Autodesk Inventor part; units mm, degrees
ref_plane "YZ Plane" through (0, 0, 0) normal (1, 0, 0) x (0, 1, 0)
ref_plane "XZ Plane" through (0, 0, 0) normal (0, 1, 0) x (-1, 0, 0)
ref_plane "XY Plane" through (0, 0, 0) normal (0, 0, 1) x (1, 0, 0)
sketch "Sketch1" plane through (0, 0, 0) normal (0, 1, 0) x (-1, 0, 0)
  line L0 (-57.5, 21.5) -> (57.5, 21.5)
  line L1 (57.5, 21.5) -> (57.5, -21.5)
  line L2 (57.5, -21.5) -> (-57.5, -21.5)
  line L3 (-57.5, -21.5) -> (-57.5, 21.5)
  line L4 (-57.5, 21.5) -> (57.5, -21.5) construction
  line L5 (57.5, 21.5) -> (-57.5, -21.5) construction
  point P0 (0, 0)
  dimension "d0" = 115
  dimension "d1" = 43
extrude "Extrusion1" add sketch "Sketch1" along normal blind 1.6
sketch "Sketch2" plane through (0, 1.6, 0) normal (0, 1, 0) x (1, 0, 0)
  line L0 (57.5, 21.5) -> (-57.5, 21.5)
  line L1 (57.5, 21.5) -> (54.5, 21.5)
  line L2 (57.5, -21.5) -> (57.5, 21.5)
  line L3 (54.5, 21.5) -> (57.5, 21.5)
  line L4 (57.5, 21.5) -> (57.5, 18.5)
  line L5 (57.5, 18.5) -> (54.5, 21.5)
  point P0 (0, 0)
  dimension "d4" = 3
  dimension "d5" = 3
extrude "Extrusion2" cut sketch "Sketch2" against normal blind 1.6
sketch "Sketch3" plane through (0, 1.6, 0) normal (0, 1, 0) x (1, 0, 0)
  line L0 (57.5, -21.5) -> (57.5, 18.5)
  circle A0 centre (53.5, 17.5) radius 1.5
  point P0 (0, 0)
  dimension "d11" = 3
extrude "Extrusion3" cut sketch "Sketch3" against normal blind 1.6
sketch "Sketch4" plane through (0, 1.6, 0) normal (0, 1, 0) x (1, 0, 0)
  line L0 (-57.5, 21.5) -> (-57.5, -21.5)
  line L1 (-57.5, 15) -> (-49.5, 15)
  line L2 (-49.5, 15) -> (-49.5, 18.5)
  line L3 (54.5, 21.5) -> (-57.5, 21.5)
  line L4 (-46.5, 21.5) -> (-49.5, 18.5)
  circle A0 centre (-45.5, 18) radius 1.5
  point P0 (0, 0)
  dimension "d15" = 8
  dimension "d16" = 3.5
  dimension "d20" = 3
extrude "Extrusion4" cut sketch "Sketch4" against normal blind 1.6 contours L3 L4 L2 L1 L0
sketch "Sketch5" plane through (0, 1.6, 0) normal (0, 1, 0) x (1, 0, 0)
  line L0 (54.5, 21.5) -> (-46.5, 21.5)
  circle A0 centre (-45.5, 17.5) radius 1.5
  point P0 (0, 0)
  dimension "d25" = 3
extrude "Extrusion5" cut sketch "Sketch5" against normal blind 1.6
mirror "Mirror1" about plane through (0, 0, 0) normal (0, 0, 1) of "Extrusion4", "Extrusion5", "Extrusion2"
sketch "Sketch7" plane through (0, 1.6, 0) normal (0, 1, 0) x (1, 0, 0)
  line L0 (-54.4988, 14.0073) -> (-26.4988, 14.0073)
  line L1 (-26.4988, 14.0073) -> (-26.4988, -13.9927)
  line L2 (-26.4988, -13.9927) -> (-54.4988, -13.9927)
  line L3 (-54.4988, -13.9927) -> (-54.4988, 14.0073)
  point P0 (0, 0)
  dimension "d30" = 28
  dimension "d31" = 28
extrude "Extrusion6" add sketch "Sketch7" along normal blind 14
sketch "Sketch8" plane through (0, 15.6, 0) normal (0, 1, 0) x (1, 0, 0)
  line L0 (-26.4988, 14.0073) -> (-26.4988, -13.9927)
  line L1 (-26.4988, 14.0073) -> (-36.4988, 14.0073)
  line L2 (-54.4988, 14.0073) -> (-26.4988, 14.0073)
  line L3 (-36.4988, 14.0073) -> (-37.9988, 14.0073)
  line L4 (-37.9988, 14.0073) -> (-36.4988, 14.0073)
  line L5 (-36.4988, 14.0073) -> (-36.4988, 12.5073)
  line L6 (-36.4988, 12.5073) -> (-48.9988, 12.5073)
  line L7 (-48.9988, 12.5073) -> (-48.9988, -12.4927)
  line L8 (-48.9988, -12.4927) -> (-36.4988, -12.4927)
  line L9 (-36.4988, -12.4927) -> (-36.4988, 12.5073)
  point P0 (0, 0)
  dimension "d34" = 10
  dimension "d35" = 1.5
  dimension "d36" = 1.5
  dimension "d37" = 12.5
  dimension "d38" = 25
extrude "Extrusion7" add sketch "Sketch8" along normal blind 0.2
sketch "Sketch9" plane through (0, 1.6, 0) normal (0, 1, 0) x (1, 0, 0)
  line L0 (-57.5, 15) -> (-57.5, -15)
  line L1 (-57.5, 15) -> (-23.75, 15)
  line L2 (-23.75, 15) -> (-23.75, 5.25)
  line L3 (-23.75, 5.25) -> (-13.25, 5.25)
  line L4 (-13.25, 5.25) -> (-13.25, -5.25)
  line L5 (-13.25, -5.25) -> (-23.75, -5.25)
  line L6 (-23.75, -5.25) -> (-23.75, 5.25)
  point P0 (0, 0)
  dimension "d41" = 33.75
  dimension "d43" = 9.75
  dimension "d44" = 10.5
  dimension "d45" = 10.5
extrude "Extrusion8" add sketch "Sketch9" along normal blind 14
sketch "Sketch10" plane through (0, 15.6, 0) normal (0, 1, 0) x (1, 0, 0)
  circle A0 centre (-18.5, 0) radius 6.25
  point P0 (0, 0)
  dimension "d48" = 12.5
extrude "Extrusion9" add sketch "Sketch10" along normal blind 3.5
sketch "Sketch11" plane through (0, 1.6, 0) normal (0, 1, 0) x (1, 0, 0)
  line L0 (54.5, -21.5) -> (57.5, -18.5)
  line L1 (57.5, -18.5) -> (55.85, -18.5)
  line L2 (55.85, -18.5) -> (55.85, -16.4)
  line L3 (55.85, -16.4) -> (57.5, -16.4)
  line L4 (57.5, -16.4) -> (57.5, -18.5)
  line L5 (55.85, -16.4) -> (-10.35, -16.4)
  line L6 (-10.35, -16.4) -> (-10.35, 3.2)
  line L7 (-10.35, 3.2) -> (55.85, 3.2)
  line L8 (55.85, 3.2) -> (55.85, -16.4)
  point P0 (0, 0)
  dimension "d51" = 1.65
  dimension "d52" = 2.1
  dimension "d53" = 66.2
  dimension "d54" = 19.6
extrude "Extrusion10" add sketch "Sketch11" along normal blind 16 contours L5 L6 L7 L8
sketch "Sketch12" plane through (0, 0, 0) normal (0, -1, 0) x (1, 0, 0)
  line L0 (57.5, 18.5) -> (57.5, -18.5)
  line L1 (57.5, -18.5) -> (57.5, -8.5)
  line L2 (57.5, -8.5) -> (48.2, -8.5)
  line L3 (48.2, -8.5) -> (48.2, 9)
  line L4 (48.2, 9) -> (57.5, 9)
  line L5 (57.5, 9) -> (57.5, -8.5)
  point P0 (0, 0)
  dimension "d57" = 10
  dimension "d58" = 9.3
  dimension "d59" = 17.5
extrude "Extrusion11" add sketch "Sketch12" along normal blind 16
sketch "Sketch13" plane through (0, 0, 0) normal (0, -1, 0) x (1, 0, 0)
  line L0 (57.5, -8.5) -> (48.2, -8.5)
  line L1 (48.2, -8.5) -> (48.2, -16)
  line L2 (48.2, -16) -> (24, -16)
  line L3 (24, -16) -> (24, 9)
  line L4 (24, 9) -> (48.2, 9)
  line L5 (48.2, 9) -> (48.2, -16)
  line L6 (24, -16) -> (24, -20)
  line L7 (54.5, -21.5) -> (-46.5, -21.5)
  line L8 (24, -20) -> (9, -20)
  line L9 (24, 9) -> (24, 10)
  line L10 (24, 10) -> (9, 10)
  line L11 (9, 10) -> (9, -20)
  line L12 (9, -20) -> (24, -20)
  line L13 (24, -20) -> (24, 10)
  point P0 (0, 0)
  dimension "d62" = 7.5
  dimension "d63" = 24.2
  dimension "d64" = 25
  dimension "d65" = 4
  dimension "d66" = 15
  dimension "d67" = 1
extrude "Extrusion12" add sketch "Sketch13" along normal blind 16 contours L1 L2 L3 L4 L5
sketch "Sketch14" plane through (0, 0, 0) normal (0, -1, 0) x (1, 0, 0)
  line L0 (24, -16) -> (24, 9)
  line L1 (24, -16) -> (24, -20)
  line L2 (24, -20) -> (9, -20)
  line L3 (24, 9) -> (24, 10)
  line L4 (24, 10) -> (9, 10)
  line L5 (9, 10) -> (9, -20)
  line L6 (9, -20) -> (24, -20)
  line L7 (24, -20) -> (24, 10)
  point P0 (0, 0)
  dimension "d70" = 4
  dimension "d71" = 15
  dimension "d72" = 1
extrude "Extrusion13" add sketch "Sketch14" along normal blind 27
properties part number "teaser_PCB"
Verification items for the finished model (mm, model axes). A direction names the side the tool comes from. Round coordinates to 2 decimals unless told otherwise and drop trailing zeros. Write each loop counter-clockwise with the first axis right and the second up, starting at its lowest first coordinate (ties: lowest second). Pieces come first, ordered by that corner, then holes. Notation, with made-up numbers: (19, 46.25) -> (44, 46.25) arc R27 cw to (44, 85.25) -> close; hole circle Ø3 at (18, -5). An arc over 180 degrees is marked (long way). Write each question's results on one line, items separated by ' | '.
Q1. Sectioned sample at D-D, the plane x = 38. Record the boundary of the cut face in (y, z), and give its area (3 significant figures).
Derived:
outline: (-16, -16) -> (0, -16) -> (0, -21.5) -> (1.6, -21.5) -> (1.6, -3.2) -> (17.6, -3.2) -> (17.6, 16.4) -> (1.6, 16.4) -> (1.6, 21.5) -> (0, 21.5) -> (0, 9) -> (-16, 9) -> close | area: 782 mm²
Q2. Thickness scan on probe 1 along X at (y, z) = (1.1, -17.5); probe 2 along Z at (x, y) = (-45.5, 0.4); probe 3 along Z at (x, y) = (53.5, 0.75). Record the ranges inside material, lowest first.
Derived:
probe 1: x = -49.5 to -47, -44 to 52, 55 to 57.5 | probe 2: z = -21.5 to -19, -16 to 16, 19 to 21.5 | probe 3: z = -21.5 to -19, -16 to 21.5
Q3. Sectioned sample at B-B, the plane y = 4. Record the boundary of the cut face in (x, z), and give its area (3 significant figures).
Derived:
outline: (-54.5, -14.01) -> (-26.5, -14.01) -> (-26.5, 13.99) -> (-54.5, 13.99) -> close; (-23.75, -5.25) -> (-13.25, -5.25) -> (-13.25, 5.25) -> (-23.75, 5.25) -> close; (-10.35, -3.2) -> (55.85, -3.2) -> (55.85, 16.4) -> (-10.35, 16.4) -> close | area: 2,190 mm²
Q4. Access from +Z, -Z, +X, -X, +Y, -Y to the whole of each face (thin tool, end or side, straight path). Record for faces 1 (the face through (-23.46, 17.33, -3.8)), 2 (the face through (36, -8, -16)), 3 (the face through (-40, 9, 13.993)).
Derived:
face 1: +Y | face 2: -Z, +X, -Y | face 3: +Z, -X, +Y
Q5. Draft check along X on faces 4 (the face through (-18, 9, 5.25)), 5 (the face through (-19, 9, -5.25)), 6 (the face through (56, 1, 20)). Enter one of: released by +X, released by -X, zero draft, split by the parting line, or undercut.
Derived:
face 4: undercut | face 5: zero draft | face 6: released by +X
Q6. Go/stop test with flat-tipped pins: pin 1 Ø13.5 at (y, z) = (-7, -5) entering from -X; pin 2 Ø2 at (y, z) = (-6, -11) entering from +X; pin 3 Ø8 at (x, z) = (31, 11.5) entering from -Y. Record where each tip stops, or that it passes through.
Derived:
pin 1: stops at x = 9 | pin 2: stops at x = 48.2 | pin 3: stops at y = -16
Q7. Sectioned sample at C-C, the plane x = -1. Record the boundary of the cut face in (y, z), and give its area (3 significant figures).
Derived:
outline: (0, -21.5) -> (1.6, -21.5) -> (1.6, -3.2) -> (17.6, -3.2) -> (17.6, 16.4) -> (1.6, 16.4) -> (1.6, 21.5) -> (0, 21.5) -> close | area: 382 mm²
Q8. Sectioned sample at A-A, the plane z = 0. Record the boundary of the cut face in (x, y).
Derived:
outline: (-57.5, 0) -> (9, 0) -> (9, -27) -> (24, -27) -> (24, -16) -> (57.5, -16) -> (57.5, 1.6) -> (55.85, 1.6) -> (55.85, 17.6) -> (-10.35, 17.6) -> (-10.35, 1.6) -> (-13.25, 1.6) -> (-13.25, 15.6) -> (-12.25, 15.6) -> (-12.25, 19.1) -> (-24.75, 19.1) -> (-24.75, 15.6) -> (-23.75, 15.6) -> (-23.75, 1.6) -> (-26.5, 1.6) -> (-26.5, 15.6) -> (-36.5, 15.6) -> (-36.5, 15.8) -> (-49, 15.8) -> (-49, 15.6) -> (-54.5, 15.6) -> (-54.5, 1.6) -> (-57.5, 1.6) -> close
